For this review, take the finished solid that the model builds, in its own axes (mm). Face numbers are marked on the shaded views. A direction names the side the tool comes from. Coordinates: 2 decimals unless noted, no trailing zeros. Loops run counter-clockwise (first coordinate to the right, second up) from the corner with the lowest first, then second, coordinate; pieces in that order, holes last. Notation, with made-up numbers: M 2.25,83 L 10.25,83 A23 cw 10.25,106 Z; hole C 66.5,28 d7. An arc over 180 degrees is marked long. Answer as a JSON object with one key per item and string values. Group by question number.
Item 1: Mouldability with a two-part tool opening along X and no side actions: class the marked faces 3, 4 and 5 as +X half, -X half, draft (parallel to the pull), parting line (faces both ways), or undercut.
Item 2: Tool access review of the marked faces 1 and 2: name each direction out of +Z, -Z, +X, -X, +Y, -Y from which nothing blocks a thin tool from reaching the whole face with its end or side.
Item 3: Wall thickness on L1, parallel to Z at x = 14, y = 5.75; L2, parallel to X at y = 12.25, z = 5.75; L3, parallel to X at y = 8.75, z = 2.25: over which ranges is each line inside the solid? List them lowest first. Write a range as from..to.
Item 4: Add section C-C (z = 5). State the section outline as (x, y) points.
Item 5: Add section D-D (z = 2.5). State the section outline as (x, y) points, then the cut area to 3 significant figures.
Item 6: Add section A-A (x = 14). State the section outline as (y, z) points, then the cut area to 3 significant figures.
Item 7: Insertion check: pin 1 (3.5 mm diameter, centred on y = 16.5, z = 6, fed in from -X); pin 2 (1.5 mm diameter, centred on x = 8.5, z = 9, fed in from +Y). Each pin has a flat end and moves straight along its axis. Give the tip position at first contact, or say it passes through.
Item 8: Add section B-B (y = 11.5). State the section outline as (x, z) points, then the cut area to 3 significant figures.
Autodesk Inventor part; units mm, degrees
ref_plane "YZ Plane" through (0, 0, 0) normal (1, 0, 0) x (0, 1, 0)
ref_plane "XZ Plane" through (0, 0, 0) normal (0, 1, 0) x (-1, 0, 0)
ref_plane "XY Plane" through (0, 0, 0) normal (0, 0, 1) x (1, 0, 0)
sketch "Sketch1" plane through (0, 0, 0) normal (0, 0, 1) x (1, 0, 0)
  line L0 (0, 0) -> (0, 13)
  line L1 (0, 13) -> (10, 13)
  line L2 (10, 13) -> (10, 20)
  line L3 (10, 20) -> (20, 20)
  line L4 (20, 20) -> (20, 0)
  line L5 (20, 0) -> (0, 0)
  dimension "d0" = 20
  dimension "d2" = 20
  dimension "d3" = 10
  dimension "d4" = 7
extrude "Extrusion1" add sketch "Sketch1" along normal blind 10
sketch "Sketch2" plane through (0, 0, 0) normal (0, -1, 0) x (1, 0, 0)
  line L0 (20, 0) -> (20, 10)
  line L1 (0, 10) -> (20, 10)
  line L2 (0, 0) -> (0, 10)
  circle A0 centre (6, 5) radius 3
  circle A1 centre (14, 5) radius 3
  dimension "d7" = 6
  dimension "d9" = 6
  dimension "d10" = 5
  dimension "d11" = 6
  dimension "d12" = 6
extrude "Extrusion2" cut sketch "Sketch2" against normal blind 22
sketch "Sketch3" plane through (0, 0, 0) normal (0, 0, -1) x (-1, 0, 0)
  line L0 (0, 0) -> (0, 13)
  line L1 (-20, 0) -> (0, 0)
  circle A0 centre (-10, 2.5) radius 1.25
  dimension "d15" = 2.5
  dimension "d17" = 2.5
  dimension "d18" = 10
hole "Hole1" at (10, 2.5, 0) direction (0, 0, 1) diameter 2.5 depth 3 tip angle 118
thread "Thread1"
properties part number "heHeaterBlock"
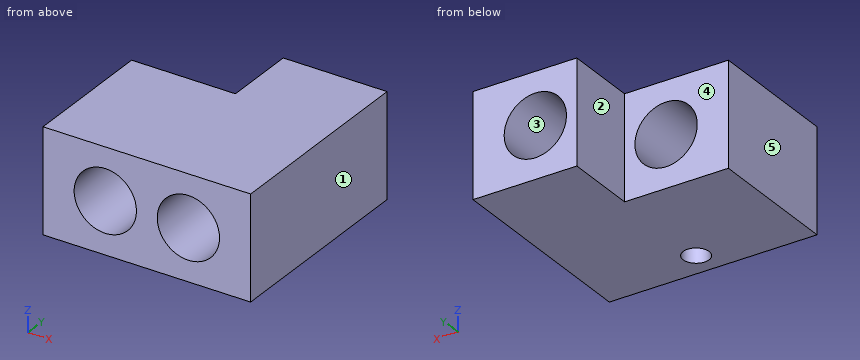
From the geometry:
{
 "1": {"face 3": "undercut", "face 4": "draft", "face 5": "-X half"},
 "2": {"face 1": "+Z, -Z, +X, +Y, -Y", "face 2": "+Z, -Z, -X, +Y"},
 "3": {"L1": "z = 0..2, 8..10", "L2": "x = 0..3.1, 8.9..11.1, 16.9..20", "L3": "x = 0..4.8, 7.2..12.8, 15.2..20"},
 "4": {"outline": "M 0,0 L 3,0 L 3,13 L 0,13 Z; M 9,0 L 11,0 L 11,20 L 10,20 L 10,13 L 9,13 Z; M 17,0 L 20,0 L 20,20 L 17,20 Z"},
 "5": {"outline": "M 0,0 L 4.34,0 L 4.34,13 L 0,13 Z; M 7.66,0 L 12.34,0 L 12.34,20 L 10,20 L 10,13 L 7.66,13 Z; M 15.66,0 L 20,0 L 20,20 L 15.66,20 Z; hole C 10,2.5 d2.5", "area": "216 mm²"},
 "6": {"outline": "M 0,0 L 20,0 L 20,2 L 0,2 Z; M 0,8 L 20,8 L 20,10 L 0,10 Z", "area": "80.0 mm²"},
 "7": {"pin 1": "stops at x = 10", "pin 2": "stops at y = 13"},
 "8": {"outline": "M 0,0 L 20,0 L 20,10 L 0,10 Z; hole C 6,5 d6; hole C 14,5 d6", "area": "143 mm²"}
}
